Check sheet for the modelled part. Datum: model origin and axes. Units: mm. Face numbers are marked on the shaded views. A direction names the side the tool comes from. Coordinates: 2 decimals unless noted, no trailing zeros. Write each loop counter-clockwise with the first axis right and the second up, starting at its lowest first coordinate (ties: lowest second). Pieces come first, ordered by that corner, then holes. Notation, with made-up numbers: M -23.75,-18.75 L 22.25,-18.75 A31 ccw 22.25,9.25 Z; hole C -27.75,84.25 d3. An arc over 180 degrees is marked long. Answer as CSV lines item,"result".
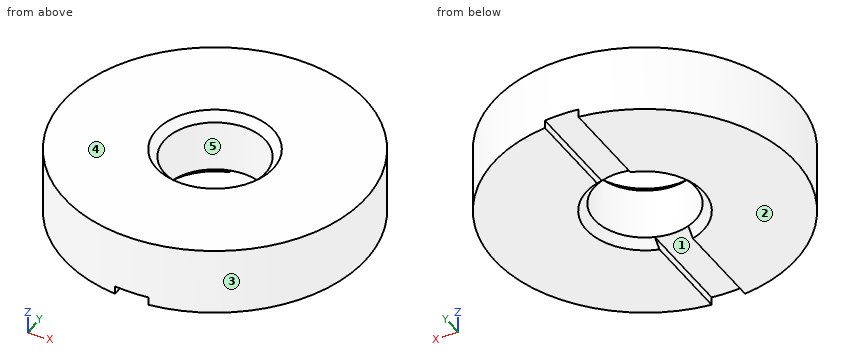
from build123d import *

# Parameters (mm, degrees)
SKETCH1_R          = 14.2875
SKETCH1_R_2        = 4.7879
EXTRUDE1_DEPTH     = 6.35
CHAMFER2_SIZE      = 0.762
SKETCH2_W          = 3.175
SKETCH2_H          = 28.575
CUT_EXTRUDE1_DEPTH = 0.762


with BuildPart() as part:
    # Sketch1 → Extrude1 (new body)
    with BuildSketch(Plane.XY):
        with Locations(Location((0, 0, 0), (0, 0, 96.379370208))):  # turned: the seam where the file's is
            Circle(SKETCH1_R)
        with Locations(Location((0, 0, 0), (0, 0, 109.363791367))):  # turned: the seam where the file's is
            Circle(SKETCH1_R_2, mode=Mode.SUBTRACT)
    extrude(amount=EXTRUDE1_DEPTH)

    # Chamfer2
    chamfer2_edges = [part.edges().sort_by_distance(p)[0] for p in [
        (1.5875, -4.517059902, 0),
        (1.5875, -4.517059902, 6.35),
    ]]
    chamfer(chamfer2_edges, length=CHAMFER2_SIZE)

    # Sketch2 → Cut-Extrude1 (cut)
    with BuildSketch(Plane(origin=(0, 0, 0), x_dir=(-1, 0, 0), z_dir=(0, 0, -1))):
        Rectangle(SKETCH2_W, SKETCH2_H)
    extrude(amount=-CUT_EXTRUDE1_DEPTH, mode=Mode.SUBTRACT)


solid = part.part
1) Thickness scan on line 1 along X through (y, z) = (0, 4.3); line 2 along Y through (x, z) = (-0.25, 4.25); line 3 along Y through (x, z) = (2.5, 2). Record the ranges inside material, lowest first.
Answer key:
line 1,"x = -14.29 to -4.79, 4.79 to 14.29"
line 2,"y = -14.29 to -4.78, 4.78 to 14.29"
line 3,"y = -14.07 to -4.08, 4.08 to 14.07"
2) Mould release check, pull along X, two halves, no side actions. Record for the marked faces 3, 4 and 5: pulls with the +X half, pulls with the -X half, needs draft (parallel to the pull), parting line crosses it, or undercut.
Answer key:
face 3,"parting line crosses it"
face 4,"needs draft"
face 5,"undercut"
3) Section check A-A, the plane x = 0. Record the boundary of the cut face in (y, z).
Answer key:
outline,"M -14.29,0.76 L -4.79,0.76 L -4.79,5.59 L -5.55,6.35 L -14.29,6.35 Z; M 4.79,0.76 L 14.29,0.76 L 14.29,6.35 L 5.55,6.35 L 4.79,5.59 Z"
4) Depth check by flat-ended pin: P1, Ø0.6, axis at y = 10.5, z = 0.5, coming from the +X side; P2, Ø1, axis at x = 0.5, y = -9.5, coming from the -Z side; P3, Ø0.8, axis at y = -8.5, z = 0.5, coming from the +X side. Enter the tip coordinate at first touch or a pass-through.
Answer key:
P1,"stops at x = 10"
P2,"stops at z = 0.76"
P3,"stops at x = 11.77"
5) Section check B-B, the plane y = 0. Record the boundary of the cut face in (x, z).
Answer key:
outline,"M -14.29,0 L -5.55,0 L -4.79,0.76 L -4.79,5.59 L -5.55,6.35 L -14.29,6.35 Z; M 4.79,0.76 L 5.55,0 L 14.29,0 L 14.29,6.35 L 5.55,6.35 L 4.79,5.59 Z"
6) Section check C-C, the plane z = 4.5. Record the boundary of the cut face in (x, y) (1 decimal).
Answer key:
outline,"C 0,0 d28.6; hole C 0,0 d9.6"
7) Section check D-D, the plane y = -8.25. Record the boundary of the cut face in (x, z), plus the area to 3 significant figures.
Answer key:
outline,"M -11.66,0 L -1.59,0 L -1.59,0.76 L 1.59,0.76 L 1.59,0 L 11.66,0 L 11.66,6.35 L -11.66,6.35 Z"
area,"146 mm2"
8) Tool access check on the marked faces 1 and 2. Record the directions out of +Z, -Z, +X, -X, +Y, -Y that give a thin tool (end or side, any length) a straight path to the whole face; none if there is none.
Answer key:
face 1,"-Z, +Y, -Y"
face 2,"-Z, +X, -X, +Y, -Y"
